Here's the drawing with two shaded views (mm, measured from the low corner). I have some questions. Round coordinates to 2 decimals unless told otherwise and drop trailing zeros. Order: outer loops, then holes, each group sorted by start corner. A loop starts at its lowest first (then second) coordinate and runs counter-clockwise, first axis right, second up. Notation, with made-up numbers: (-7, -12) -> (48, -12) arc R4 ccw to (48, -5) -> close; hole circle Ø8 at (10.25, 86.5). An arc over 180 degrees is marked (long way). Answer in a Markdown table with one row per item.
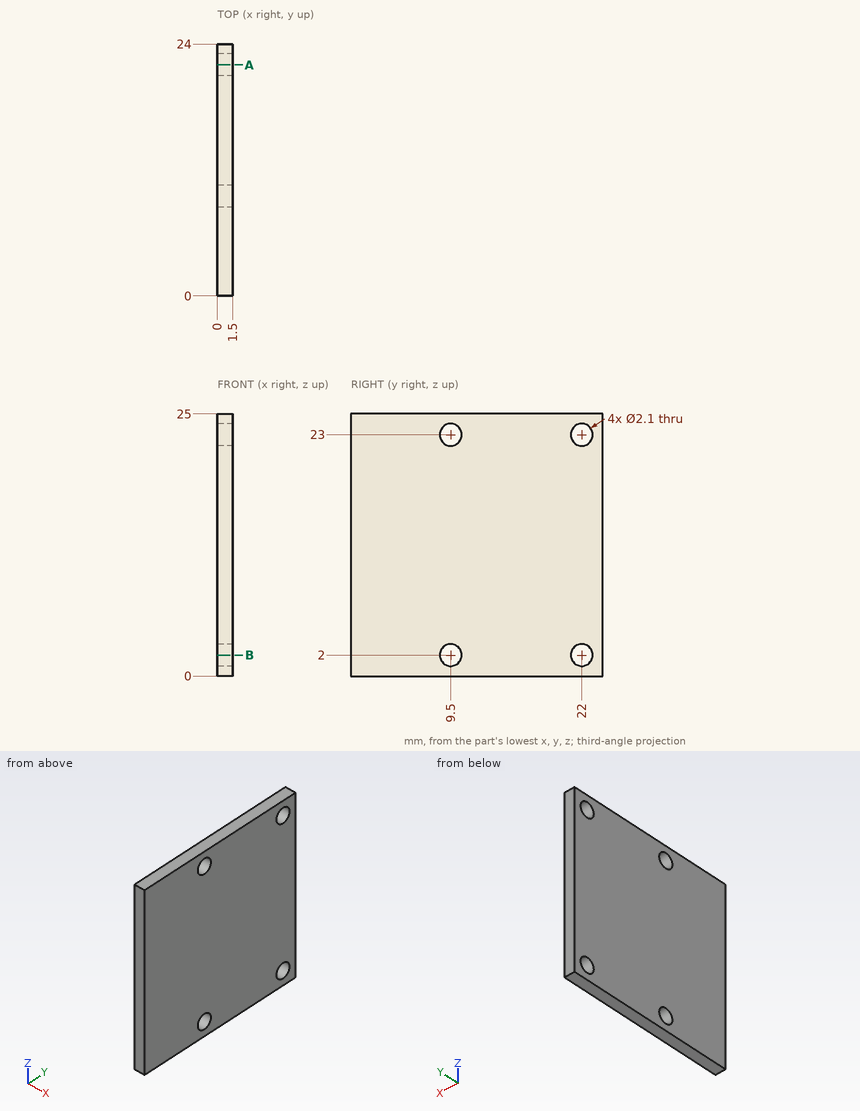
1. Please list where these lines run through material, in increasing order: line 1 along Z through (x, y) = (0.8, 9.5); line 2 along Z through (x, y) = (1.1, 9); line 3 along Y through (x, z) = (0.15, 2.25).
Numbers:
| item | result |
|---|---|
| line 1 | z = 0 to 0.95, 3.05 to 21.95, 24.05 to 25 |
| line 2 | z = 0 to 1.08, 2.92 to 22.08, 23.92 to 25 |
| line 3 | y = 0 to 8.48, 10.52 to 20.98, 23.02 to 24 |
2. For pin 1 Ø1.7 at (y, z) = (22, 2) entering from -X, with a flat end and sliding along its axis, tell me the tip position at first contact or that it passes through.
Numbers:
| item | result |
|---|---|
| pin 1 | passes through |
3. Suppose I cut it at B-B on z = 2. Write out the boundary of the cut face in (x, y), then the cut area to 3 significant figures.
Numbers:
| item | result |
|---|---|
| outline | (0, 0) -> (1.5, 0) -> (1.5, 8.45) -> (0, 8.45) -> close; (0, 10.55) -> (1.5, 10.55) -> (1.5, 20.95) -> (0, 20.95) -> close; (0, 23.05) -> (1.5, 23.05) -> (1.5, 24) -> (0, 24) -> close |
| area | 29.7 mm2 |
4. Suppose I cut it at A-A on y = 22. Write out the boundary of the cut face in (x, z).
Numbers:
| item | result |
|---|---|
| outline | (0, 0) -> (1.5, 0) -> (1.5, 0.95) -> (0, 0.95) -> close; (0, 3.05) -> (1.5, 3.05) -> (1.5, 21.95) -> (0, 21.95) -> close; (0, 24.05) -> (1.5, 24.05) -> (1.5, 25) -> (0, 25) -> close |
